```python
from build123d import *

# Parameters (mm, degrees)
SKETCH_1_R          = 10
SKETCH_1_R_2        = 4
EXTRUDE_1_DEPTH     = 23
CHAMFER_1_SIZE      = 0.5
SKETCH_2_W          = 20
SKETCH_2_H          = 23
CUT_EXTRUDE_1_DEPTH = 23
SKETCH_3_R          = 1.5
CUT_EXTRUDE_2_DEPTH = 29.022312538


with BuildPart() as part:
    # 草图1 → 凸台-拉伸1 (new body)
    with BuildSketch(Plane(origin=(0, 0, 0), x_dir=(1, 0, 0), z_dir=(0, 1, 0))):
        with Locations(Location((0, 0, 0), (0, 0, 270))):
            Circle(SKETCH_1_R)
        with Locations(Location((0, 0, 0), (0, 0, 270))):
            Circle(SKETCH_1_R_2, mode=Mode.SUBTRACT)
    extrude(amount=EXTRUDE_1_DEPTH)

    # 倒角1
    chamfer_1_edges = [part.edges().sort_by_distance(p)[0] for p in [
        (0, 0, -10),
        (0, 23, -10),
        (0, 0, -4),
        (0, 23, -4),
    ]]
    chamfer(chamfer_1_edges, length=CHAMFER_1_SIZE)

    # 草图2 → 切除-拉伸1 (cut)
    with BuildSketch(Plane.XY.offset(2.5)):
        with Locations((0, 11.5)):
            Rectangle(SKETCH_2_W, SKETCH_2_H)
    extrude(amount=CUT_EXTRUDE_1_DEPTH, mode=Mode.SUBTRACT)

    # 草图3 → 切除-拉伸2 (cut, through all)
    with BuildSketch(Plane.XY.offset(2.5)):
        with Locations((-6.5, 11.5)):
            Circle(SKETCH_3_R)
        with Locations((-6.5, 4)):
            Circle(SKETCH_3_R)
        with Locations((-6.5, 19)):
            Circle(SKETCH_3_R)
        with Locations((6.5, 19)):
            Circle(SKETCH_3_R)
        with Locations((6.5, 4)):
            Circle(SKETCH_3_R)
        with Locations((6.5, 11.5)):
            Circle(SKETCH_3_R)
    extrude(amount=-CUT_EXTRUDE_2_DEPTH, mode=Mode.SUBTRACT)


solid = part.part
```
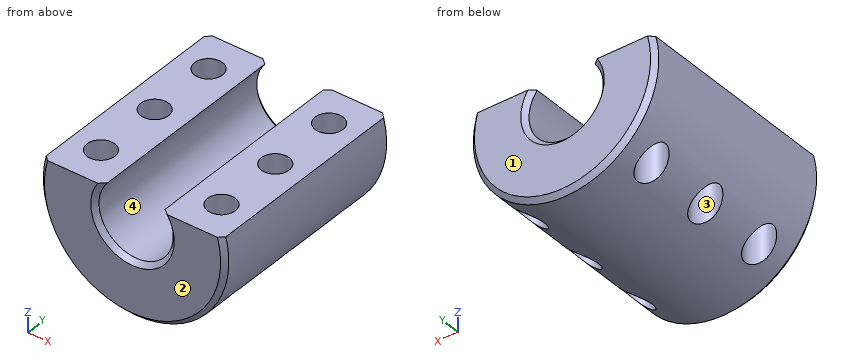
Geometry check sheet. Reference: the model listing, model coordinates, mm. Face numbers are marked on the shaded views. Give positions to 0.01 mm unless a question says otherwise; leave off trailing zeros. Order: outer loops, then holes, each group sorted by start corner. A loop starts at its lowest first (then second) coordinate and runs counter-clockwise, first axis right, second up. Notation, with made-up numbers: (-10, -23.5) -> (11, -23.5) arc R21 ccw to (11, -0.5) -> close; hole circle Ø3 at (11, -27.5). An arc over 180 degrees is marked (long way). Write each question's results on one line, items separated by ' | '. Start each with the question number.
(1) Gauge pin test, flat ends, axial feed: P1, Ø3.5, axis at x = 6.5, y = 11.5, coming from the -Z side; P2, Ø1, axis at x = 6, y = 10, coming from the -Z side; P3, Ø1.5, axis at y = 19, z = -1, coming from the +X side. Record the tip position at first contact, or that the pin passes through.
(2) Mould release check, pull along Y, two halves, no side actions. Record for the marked faces 1, 2, 3 and 4: pulls with the +Y half, pulls with the -Y half, needs draft (parallel to the pull), parting line crosses it, or undercut.
(3) Sectioned sample at A-A (y = 19). Enter the section's corners in (x, z), plus the area to 3 significant figures.
(4) Sectioned sample at B-B (z = 0). Enter the section's corners in (x, y).
(5) Sectioned sample at D-D (y = 11). Enter the section's corners in (x, z), plus the area to 3 significant figures.
(6) Scan lines: line 1 (Y direction, x = 6.5, z = -4); line 2 (X direction, y = 20, z = -4.25); line 3 (X direction, y = 20, z = -2). Record each from-to range of solid material in increasing order.
(7) Sectioned sample at C-C (x = -6.5). Give the number of separate pieces and of enclosed holes in the cut face, plus the area to 3 significant figures.
Answer below:
1) P1: z = -8.8 | P2: z = -8.35 | P3: x = 10
2) face 1: pulls with the +Y half | face 2: pulls with the -Y half | face 3: undercut | face 4: needs draft
3) outline: (-9.68, 2.5) arc R10 ccw to (-8, -6) -> (-8, 2.5) -> close; (-5, -8.66) arc R10 ccw to (5, -8.66) -> (5, 2.5) -> (3.12, 2.5) arc R4 cw (long way) to (-3.12, 2.5) -> (-5, 2.5) -> close; (8, -6) arc R10 ccw to (9.68, 2.5) -> (8, 2.5) -> close | area: 103 mm2
4) outline: (-10, 0.5) -> (-9.5, 0) -> (-4.5, 0) -> (-4, 0.5) -> (-4, 22.5) -> (-4.5, 23) -> (-9.5, 23) -> (-10, 22.5) -> close; (4, 0.5) -> (4.5, 0) -> (9.5, 0) -> (10, 0.5) -> (10, 22.5) -> (9.5, 23) -> (4.5, 23) -> (4, 22.5) -> close; hole circle Ø3 at (-6.5, 4); hole circle Ø3 at (-6.5, 11.5); hole circle Ø3 at (-6.5, 19); hole circle Ø3 at (6.5, 4); hole circle Ø3 at (6.5, 11.5); hole circle Ø3 at (6.5, 19)
5) outline: (-9.68, 2.5) arc R10 ccw to (-7.91, -6.11) -> (-7.91, 2.5) -> close; (-5.09, -8.61) arc R10 ccw to (5.09, -8.61) -> (5.09, 2.5) -> (3.12, 2.5) arc R4 cw (long way) to (-3.12, 2.5) -> (-5.09, 2.5) -> close; (7.91, -6.11) arc R10 ccw to (9.68, 2.5) -> (7.91, 2.5) -> close | area: 106 mm2
6) line 1: 0 to 2.5, 5.5 to 10, 13 to 17.5, 20.5 to 23 | line 2: -9.05 to -7.62, -5.38 to 5.38, 7.62 to 9.05 | line 3: -9.8 to -7.62, -5.38 to -3.46, 3.46 to 5.38, 7.62 to 9.8
7) separate pieces: 4 | enclosed holes: 0 | area: 141 mm2
